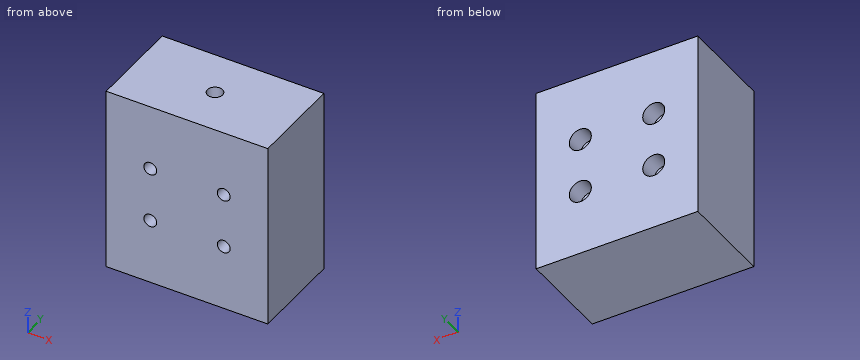
Autodesk Inventor part; units mm, degrees
ref_plane "YZ Plane" through (0, 0, 0) normal (1, 0, 0) x (0, 1, 0)
ref_plane "XZ Plane" through (0, 0, 0) normal (0, 1, 0) x (-1, 0, 0)
ref_plane "XY Plane" through (0, 0, 0) normal (0, 0, 1) x (1, 0, 0)
sketch "Sketch2" plane through (0, 0, 0) normal (0, 1, 0) x (-1, 0, 0)
  line L0 (-22, 25.4) -> (22, 25.4)
  line L1 (22, 25.4) -> (22, -25.4)
  line L2 (22, -25.4) -> (-22, -25.4)
  line L3 (-22, -25.4) -> (-22, 25.4)
  line L4 (-22, 25.4) -> (22, -25.4) construction
  line L5 (22, 25.4) -> (-22, -25.4) construction
  point P0 (0, 0)
  dimension "d0" = 50.8
  dimension "d1" = 44
extrude "Extrusion1" add sketch "Sketch2" along normal blind 25.4
sketch "Sketch3" plane through (-22, 0, 25.4) normal (0, 0, 1) x (1, 0, 0)
  line L0 (0, 25.4) -> (44, 25.4) construction
  line L1 (0, 0) -> (44, 0) construction
  line L2 (44, 0) -> (44, 25.4) construction
  line L3 (44, 25.4) -> (0, 25.4) construction
  line L4 (0, 25.4) -> (0, 0) construction
  line L5 (0, 0) -> (44, 25.4) construction
  line L6 (44, 0) -> (0, 25.4) construction
  point P0 (22, 0)
  point P1 (22, 12.7)
hole "Hole1" at (0, 12.7, 25.4) direction (0, 0, -1) diameter 4.134 depth 19.05 tip angle 118
sketch "Sketch4" plane through (0, 25.4, 0) normal (0, 1, 0) x (1, 0, 0)
  line L0 (10, -7.5) -> (10, 7.5) construction
  line L1 (10, 7.5) -> (-10, 7.5) construction
  line L2 (-10, 7.5) -> (-10, -7.5) construction
  line L3 (-10, -7.5) -> (10, -7.5) construction
  line L4 (10, -7.5) -> (-10, 7.5) construction
  line L5 (10, 7.5) -> (-10, -7.5) construction
  circle A0 centre (-10, 7.5) radius 3
  circle A1 centre (10, 7.5) radius 3
  circle A2 centre (10, -7.5) radius 3
  circle A3 centre (-10, -7.5) radius 3
  point P0 (0, 0)
  dimension "d15" = 20
  dimension "d16" = 15
  dimension "d14" = 6
  dimension "d13" = 6
  dimension "d12" = 6
  dimension "d11" = 6
extrude "Extrusion2" cut sketch "Sketch4" against normal blind 5
sketch "Sketch5" plane through (-10, 20.4, 7.5) normal (0, 1, 0) x (1, 0, 0)
  circle A0 centre (0, 15) radius 3
  circle A1 centre (20, 0) radius 3
  circle A2 centre (20, 15) radius 3
  point P0 (16, 18)
  point P1 (0, 0)
hole "Hole2" at (-10, 20.4, -7.5) at (-10, 20.4, 7.5) at (10, 20.4, 7.5) at (10, 20.4, -7.5) direction (0, -1, 0) diameter 3.5 end through all
properties part number "Mass 3" material "Steel, Mild"
Input: part model. Units: mm. Frame: model coordinates. Give positions to 0.01 mm unless a question says otherwise; leave off trailing zeros. Loops run counter-clockwise (first coordinate to the right, second up) from the corner with the lowest first, then second, coordinate; pieces in that order, holes last. Notation, with made-up numbers: (-34, -15.75) -> (-26, -15.75) arc R31 ccw to (-26, 9.25) -> close; hole circle Ø10 at (84, -10.5). An arc over 180 degrees is marked (long way). Use a Markdown table: item, result.
Q1. First-contact query: P1, Ø4.5, axis at x = -10, z = -7.5, coming from the +Y side; P2, Ø5, axis at x = -16, z = -17, coming from the -Y side; P3, Ø3, axis at x = -10, z = 7.5, coming from the +Y side. Flat tips, straight axial feed; report the tip coordinate or a pass-through.
Entries:
| item | result |
|---|---|
| P1 | stops at y = 20.4 |
| P2 | stops at y = 0 |
| P3 | passes through |
Q2. Section query D-D, the plane x = 9. Return the cut outline in (y, z), plus the area to 3 significant figures.
Entries:
| item | result |
|---|---|
| outline | (0, -25.4) -> (25.4, -25.4) -> (25.4, -10.33) -> (20.4, -10.33) -> (20.4, -8.94) -> (0, -8.94) -> close; (0, -6.06) -> (20.4, -6.06) -> (20.4, -4.67) -> (25.4, -4.67) -> (25.4, 4.67) -> (20.4, 4.67) -> (20.4, 6.06) -> (0, 6.06) -> close; (0, 8.94) -> (20.4, 8.94) -> (20.4, 10.33) -> (25.4, 10.33) -> (25.4, 25.4) -> (0, 25.4) -> close |
| area | 1,120 mm² |
Q3. Section query A-A, the plane x = -10. Return the cut outline in (y, z), plus the area to 3 significant figures.
Entries:
| item | result |
|---|---|
| outline | (0, -25.4) -> (25.4, -25.4) -> (25.4, -10.5) -> (20.4, -10.5) -> (20.4, -9.25) -> (0, -9.25) -> close; (0, -5.75) -> (20.4, -5.75) -> (20.4, -4.5) -> (25.4, -4.5) -> (25.4, 4.5) -> (20.4, 4.5) -> (20.4, 5.75) -> (0, 5.75) -> close; (0, 9.25) -> (20.4, 9.25) -> (20.4, 10.5) -> (25.4, 10.5) -> (25.4, 25.4) -> (0, 25.4) -> close |
| area | 1,090 mm² |
Q4. Ray query, probe 1 along Z at (x, y) = (-10, 5); probe 2 along X at (y, z) = (15.5, 7.5); probe 3 along Z at (x, y) = (10, 21.7). Return the intervals inside material, ascending. Write a range as from..to.
Entries:
| item | result |
|---|---|
| probe 1 | z = -25.4..-9.25, -5.75..5.75, 9.25..25.4 |
| probe 2 | x = -22..-11.75, -8.25..8.25, 11.75..22 |
| probe 3 | z = -25.4..-10.5, -4.5..4.5, 10.5..25.4 |
Q5. Section query C-C, the plane y = 4.5. Return the cut outline in (x, z).
Entries:
| item | result |
|---|---|
| outline | (-22, -25.4) -> (22, -25.4) -> (22, 25.4) -> (-22, 25.4) -> close; hole circle Ø3.5 at (-10, -7.5); hole circle Ø3.5 at (-10, 7.5); hole circle Ø3.5 at (10, -7.5); hole circle Ø3.5 at (10, 7.5) |
Q6. Section query B-B, the plane z = 7.5. Return the cut outline in (x, y).
Entries:
| item | result |
|---|---|
| outline | (-22, 0) -> (-11.75, 0) -> (-11.75, 20.4) -> (-13, 20.4) -> (-13, 25.4) -> (-22, 25.4) -> close; (-8.25, 0) -> (8.25, 0) -> (8.25, 20.4) -> (7, 20.4) -> (7, 25.4) -> (-7, 25.4) -> (-7, 20.4) -> (-8.25, 20.4) -> close; (11.75, 0) -> (22, 0) -> (22, 25.4) -> (13, 25.4) -> (13, 20.4) -> (11.75, 20.4) -> close; hole circle Ø4.13 at (0, 12.7) |
